Print and shaded views of the part. All mm, measured from the part's lowest x, y and z. A direction names the side the tool comes from. Round coordinates to 2 decimals unless told otherwise and drop trailing zeros. Write each loop counter-clockwise with the first axis right and the second up, starting at its lowest first coordinate (ties: lowest second). Pieces come first, ordered by that corner, then holes.
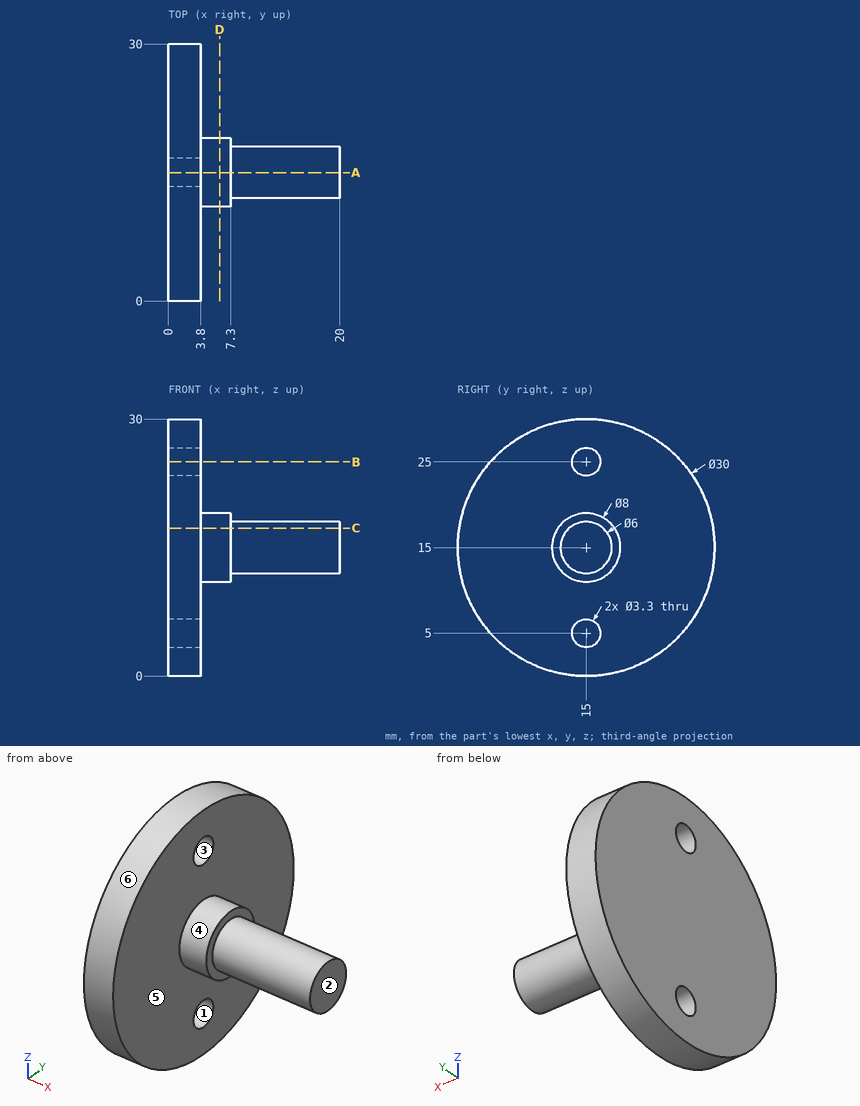
1) Mould opens along Y. For the marked faces 1, 2, 3 and 4 say: released by +Y, released by -Y, zero draft, split by the parting line, or undercut.
Results:
face 1: undercut
face 2: zero draft
face 3: undercut
face 4: split by the parting line
2) Pin check, flat tips, straight feed: pin 1 Ø10 at (x, z) = (6, 10) entering from +Y; pin 2 Ø4 at (y, z) = (11, 6.5) entering from +X; pin 3 Ø3 at (x, y) = (16.5, 13.5) entering from -Z. Stop position of each tip, or through.
Results:
pin 1: stops at y = 29.99
pin 2: stops at x = 3.8
pin 3: stops at z = 12
3) Slice it at D-D (x = 6). Write the cut outline in (y, z), plus the area to 3 significant figures.
Results:
outline: circle Ø8 at (15, 15)
area: 50.3 mm2
4) Wall check: L1, parallel to X at y = 11.75, z = 24.5; L2, parallel to Y at x = 1.3, z = 25; L3, parallel to Z at x = 3.75, y = 14.5. Give the ranges that are in metal, low to high.
Results:
L1: x = 0 to 3.8
L2: y = 3.82 to 13.35, 16.65 to 26.18
L3: z = 0.01 to 3.43, 6.57 to 23.43, 26.57 to 29.99
5) Slice it at C-C (z = 17.25). Write the cut outline in (x, y), plus the area to 3 significant figures.
Results:
outline: (0, 0.17) - (3.8, 0.17) - (3.8, 11.69) - (7.3, 11.69) - (7.3, 13.02) - (20, 13.02) - (20, 16.98) - (7.3, 16.98) - (7.3, 18.31) - (3.8, 18.31) - (3.8, 29.83) - (0, 29.83) - close
area: 186 mm2
6) Slice it at B-B (z = 25). Write the cut outline in (x, y), plus the area to 3 significant figures.
Results:
outline: (0, 3.82) - (3.8, 3.82) - (3.8, 13.35) - (0, 13.35) - close; (0, 16.65) - (3.8, 16.65) - (3.8, 26.18) - (0, 26.18) - close
area: 72.4 mm2
7) Slice it at A-A (y = 15). Write the cut outline in (x, z), plus the area to 3 significant figures.
Results:
outline: (0, 0) - (3.8, 0) - (3.8, 3.35) - (0, 3.35) - close; (0, 6.65) - (3.8, 6.65) - (3.8, 11) - (7.3, 11) - (7.3, 12) - (20, 12) - (20, 18) - (7.3, 18) - (7.3, 19) - (3.8, 19) - (3.8, 23.35) - (0, 23.35) - close; (0, 26.65) - (3.8, 26.65) - (3.8, 30) - (0, 30) - close
area: 193 mm2
8) Which spindle directions (+Z, -Z, +X, -X, +Y, -Y) get a long thin tool onto all of the face, cutting with end or side? Do the marked faces 5 and 6. Say none if no direction does.
Results:
face 5: +X
face 6: +X, -X
